```python
from build123d import *

# Parameters (mm, degrees)
SKETCH1_W           = 190.5
SKETCH1_H           = 57.15
BOSS_EXTRUDE1_DEPTH = 35.2298
SKETCH2_R           = 3.3782
CUT_EXTRUDE1_DEPTH  = 35.2298
SKETCH3_W           = 31.75
SKETCH3_H           = 31.75
SKETCH3_W_2         = 25.4
SKETCH3_H_2         = 25.4
BOSS_EXTRUDE2_DEPTH = 25.4
SKETCH4_R           = 3.3782
CUT_EXTRUDE2_DEPTH  = 54.975
SKETCH5_R           = 2.54
CUT_EXTRUDE3_DEPTH  = 35.2298
SKETCH6_R           = 4.064
CUT_EXTRUDE4_DEPTH  = 28.8798
CUT_EXTRUDE5_DEPTH  = 9.8298


with BuildPart() as part:
    # Sketch1 → Boss-Extrude1 (new body)
    with BuildSketch(Plane(origin=(0, 0, 0), x_dir=(1, 0, 0), z_dir=(0, 1, 0))):
        Rectangle(SKETCH1_W, SKETCH1_H)
    extrude(amount=BOSS_EXTRUDE1_DEPTH)

    # Sketch2 → Cut-Extrude1 (cut)
    with BuildSketch(Plane(origin=(0, 35.2298, 0), x_dir=(1, 0, 0), z_dir=(0, 1, 0))):
        with Locations((0, 3.0988)):
            Circle(SKETCH2_R)
    extrude(amount=-CUT_EXTRUDE1_DEPTH, mode=Mode.SUBTRACT)

    # Sketch3 → Boss-Extrude2 (add)
    with BuildSketch(Plane(origin=(0, 35.2298, 0), x_dir=(1, 0, 0), z_dir=(0, 1, 0))):
        with Locations((76.2, 9.525)):
            Rectangle(SKETCH3_W, SKETCH3_H)
        with Locations((76.2, 9.525)):
            Rectangle(SKETCH3_W_2, SKETCH3_H_2, mode=Mode.SUBTRACT)
    boss_extrude2 = extrude(amount=BOSS_EXTRUDE2_DEPTH)

    # Sketch4 → Cut-Extrude2 (cut, through all)
    with BuildSketch(Plane(origin=(0, 0, -25.4), x_dir=(-1, 0, 0), z_dir=(0, 0, -1))):
        with Locations((-76.2, 47.9298)):
            Circle(SKETCH4_R)
    cut_extrude2 = extrude(amount=-CUT_EXTRUDE2_DEPTH, mode=Mode.SUBTRACT)

    # Sketch5 → Cut-Extrude3 (cut)
    with BuildSketch(Plane.XZ):
        with Locations((80.645, 19.05)):
            Circle(SKETCH5_R)
        with Locations((39.243, -19.05)):
            Circle(SKETCH5_R)
    cut_extrude3 = extrude(amount=-CUT_EXTRUDE3_DEPTH, mode=Mode.SUBTRACT)

    # Sketch6 → Cut-Extrude4 (cut)
    with BuildSketch(Plane(origin=(0, 35.2298, 0), x_dir=(1, 0, 0), z_dir=(0, 1, 0))):
        with Locations((80.645, -19.05)):
            Circle(SKETCH6_R)
        with Locations((39.243, 19.05)):
            Circle(SKETCH6_R)
    cut_extrude4 = extrude(amount=-CUT_EXTRUDE4_DEPTH, mode=Mode.SUBTRACT)

    # Mirror1: Boss-Extrude2, Cut-Extrude2, Cut-Extrude3, Cut-Extrude4 across plane
    add(boss_extrude2.mirror(Plane(origin=(0, 0, 0), x_dir=(0, 0, 1), z_dir=(1, 0, 0))))
    add(cut_extrude2.mirror(Plane(origin=(0, 0, 0), x_dir=(0, 0, 1), z_dir=(1, 0, 0))), mode=Mode.SUBTRACT)
    add(cut_extrude3.mirror(Plane(origin=(0, 0, 0), x_dir=(0, 0, 1), z_dir=(1, 0, 0))), mode=Mode.SUBTRACT)
    add(cut_extrude4.mirror(Plane(origin=(0, 0, 0), x_dir=(0, 0, 1), z_dir=(1, 0, 0))), mode=Mode.SUBTRACT)

    # Sketch7 → Cut-Extrude5 (cut)
    with BuildSketch(Plane.XZ):
        Polygon((6.599113577, -3.0988), (3.299556788, 2.6162), (-3.299556788, 2.6162), (-6.599113577, -3.0988), (-3.299556788, -8.8138), (3.299556788, -8.8138), align=None)
    extrude(amount=-CUT_EXTRUDE5_DEPTH, mode=Mode.SUBTRACT)


solid = part.part
```
Geometry: final body of the model. Coordinates: model frame, mm. A direction names the side the tool comes from. Round coordinates to 2 decimals unless told otherwise and drop trailing zeros. Write each loop counter-clockwise with the first axis right and the second up, starting at its lowest first coordinate (ties: lowest second). Pieces come first, ordered by that corner, then holes.
Item 1: Section query A-A (y = 57.5). Return loops of the section in (x, z) (3 decimals), plus the area to 3 significant figures.
Item 2: Section query B-B (x = 0). Return loops of the section in (y, z) (3 decimals), plus the area to 3 significant figures.
Item 3: Mould query, pull axis X, two halves, no side actions, for faces 1 (the face through (-1, 35.23, 6)), 2 (the face through (-95.25, 17, 0)), 3 (the face through (-1, 17, -28.575)). Classes: +X half, -X half, draft (parallel to the pull), parting line (faces both ways), or undercut.
Item 4: Section query D-D (z = -13). Return loops of the section in (x, y) (3 decimals).
Item 5: Pin query (flat end, axial travel): P1, Ø12.5, axis at y = 45, z = -4.5, coming from the +X side (3 decimals); P2, Ø20.5, axis at x = 76, y = 50, coming from the -Z side; P3, Ø20.5, axis at x = 77, y = 48, coming from the +Z side. Return the tip coordinate at first contact, or that it passes through.
Item 6: Material intervals for L1, parallel to X at y = 40.5, z = 2 (3 decimals); L2, parallel to X at y = 4, z = -19; L3, parallel to X at y = 7, z = -21, sorted ascending.
Item 7: Section query C-C (y = 16.5). Return loops of the section in (x, z) (3 decimals).
Item 8: Set-up query: faces 4 (the face through (-38.91, 3.13, -16.53)), 5 (the face through (-84.52, 20.99, 17.83)), 6 (the face through (4.926, 4.846, -5.996)). Return all of +Z, -Z, +X, -X, +Y, -Y with unobstructed straight access to the full face (end or side cutting, diameter ignored); none if empty.
Completed:
1. outline: (-92.075, -25.4) - (-60.325, -25.4) - (-60.325, 6.35) - (-92.075, 6.35) - close; (60.325, -25.4) - (92.075, -25.4) - (92.075, 6.35) - (60.325, 6.35) - close; hole (-88.9, -22.225) - (-63.5, -22.225) - (-63.5, 3.175) - (-88.9, 3.175) - close; hole (63.5, -22.225) - (88.9, -22.225) - (88.9, 3.175) - (63.5, 3.175) - close
1. area: 726 mm2
2. outline: (0, -28.575) - (35.23, -28.575) - (35.23, -6.477) - (9.83, -6.477) - (9.83, -8.814) - (0, -8.814) - close; (0, 2.616) - (9.83, 2.616) - (9.83, 0.279) - (35.23, 0.279) - (35.23, 28.575) - (0, 28.575) - close
2. area: 1,730 mm2
3. face 1: undercut
3. face 2: -X half
3. face 3: draft
4. outline: (-95.25, 0) - (95.25, 0) - (95.25, 35.23) - (92.075, 35.23) - (92.075, 60.63) - (88.9, 60.63) - (88.9, 35.23) - (63.5, 35.23) - (63.5, 60.63) - (60.325, 60.63) - (60.325, 35.23) - (-60.325, 35.23) - (-60.325, 60.63) - (-63.5, 60.63) - (-63.5, 35.23) - (-88.9, 35.23) - (-88.9, 60.63) - (-92.075, 60.63) - (-92.075, 35.23) - (-95.25, 35.23) - close
5. P1: stops at x = 92.075
5. P2: stops at z = -25.4
5. P3: stops at z = 6.35
6. L1: x = -92.075 to -88.9, -63.5 to -60.325, 60.325 to 63.5, 88.9 to 92.075
6. L2: x = -95.25 to -41.78, -36.7 to 36.7, 41.78 to 95.25
6. L3: x = -95.25 to -42.81, -35.68 to 35.68, 42.81 to 95.25
7. outline: (-95.25, -28.575) - (95.25, -28.575) - (95.25, 28.575) - (-95.25, 28.575) - close; hole circle Ø8.128 at (-80.645, 19.05); hole circle Ø8.128 at (-39.243, -19.05); hole circle Ø6.756 at (0, -3.099); hole circle Ø8.128 at (39.243, -19.05); hole circle Ø8.128 at (80.645, 19.05)
8. face 4: +Y, -Y
8. face 5: +Y
8. face 6: -Y
